Geometry: final body of the model. Coordinates: model frame, mm. Face numbers are marked on the shaded views. A direction names the side the tool comes from. Round coordinates to 2 decimals unless told otherwise and drop trailing zeros. Loops run counter-clockwise (first coordinate to the right, second up) from the corner with the lowest first, then second, coordinate; pieces in that order, holes last. Notation, with made-up numbers: (-33.75, 50.5) - (-5.75, 50.5) arc R15 ccw to (-5.75, 60.5) - close; hole circle Ø3 at (83, -27.5). An arc over 180 degrees is marked (long way). Write item = value, one per line. Start each with the question number.
Item 1: Draft query along Z for the marked faces 1, 2 and 3. Return one class per face: pulls with the +Z half, pulls with the -Z half, needs draft (parallel to the pull), parting line crosses it, or undercut.
Item 2: Access query for the marked faces 4 and 5. Directions: +Z, -Z, +X, -X, +Y, -Y. A direction counts if a zero-diameter tool reaches every point of the face in a straight line with its end or side. Return the directions, or none.
Item 3: Section C-C (z = 2.5). Return loops of the section in (x, y).
Item 4: First-contact query: pin 1 (1.5 mm diameter, centred on y = 37, z = -3.5, fed in from +X); pin 2 (6.5 mm diameter, centred on y = 15, z = 3.45, fed in from -X); pin 3 (9 mm diameter, centred on x = -5, y = 27.5, fed in from +Z); pin 4 (10 mm diameter, centred on y = 32, z = -5.5, fed in from +X). Flat tips, straight axial feed; report the tip coordinate or a pass-through.
Item 5: Section D-D (z = -0.75). Return loops of the section in (x, y), plus the area to 3 significant figures.
Item 6: Section A-A (x = 21). Return loops of the section in (y, z), plus the area to 3 significant figures.
Item 7: Line query: line 1 (Z direction, x = -17, y = 10); line 2 (Y direction, x = 3, z = 2.5); line 3 (X direction, y = 39.5, z = 6.75). Output: solid intervals per line, ascending. Write a range as from..to.
Item 8: Section B-B (y = 40). Return loops of the section in (x, z).
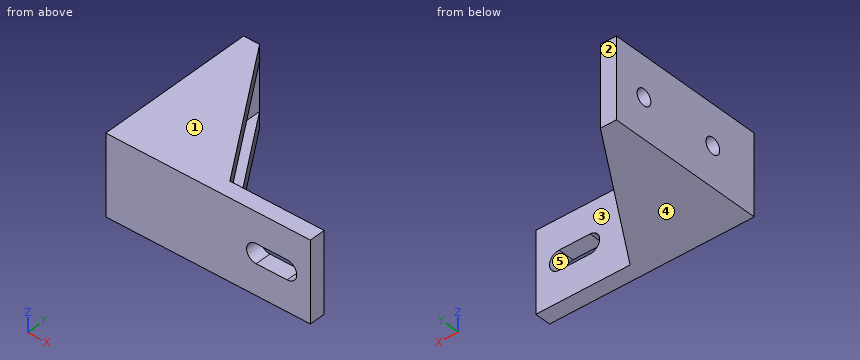
from build123d import *

# Parameters (mm, degrees)
SKETCH1_W                 = 64
SKETCH1_H                 = 15
BOSS_EXTRUDE1_DEPTH       = 5
SKETCH3_W                 = 5
SKETCH3_H                 = 15
BOSS_EXTRUDE2_DEPTH       = 45
F_5_0MM_DOWEL_HOLE1_D     = 5
F_6_0MM_DOWEL_SLOT1_DEPTH = 5
BOSS_EXTRUDE3_DEPTH       = 5
BOSS_EXTRUDE4_DEPTH       = 5


# Read off the part's stored shape, not the designer's step: Ø6.0mm Dowel Slot1
with BuildPart() as part:
    # Sketch1 → Boss-Extrude1 (new body)
    with BuildSketch(Plane(origin=(0, 0, 0), x_dir=(1, 0, 0), z_dir=(0, 1, 0))):
        with Locations((1.827783478, -3.453636176)):
            Rectangle(SKETCH1_W, SKETCH1_H)
    extrude(amount=BOSS_EXTRUDE1_DEPTH)

    # Sketch3 → Boss-Extrude2 (add)
    with BuildSketch(Plane(origin=(0, 5, 0), x_dir=(1, 0, 0), z_dir=(0, 1, 0))):
        with Locations((-27.672216522, -3.453636176)):
            Rectangle(SKETCH3_W, SKETCH3_H)
    extrude(amount=BOSS_EXTRUDE2_DEPTH)

    # Ø5.0mm Dowel Hole1 (through all)
    with Locations(Plane.ZY.offset(30.172216522)):
        with Locations((3.453636176, 15), (3.453636176, 40)):
            Hole(F_5_0MM_DOWEL_HOLE1_D / 2)

    # Ø6.0mm Dowel Slot1 outline → Ø6.0mm Dowel Slot1 (cut)
    with BuildSketch(Plane(origin=(0, 0, 0), x_dir=(1, 0, 0), z_dir=(0, 1, 0))):
        with BuildLine():
            Line((16.854220924, -6.453652479), (26.554220923, -6.453705194))
            ThreePointArc((26.554220923, -6.453705194), (29.554237227, -3.453721498), (26.554253531, -0.453705194))
            Line((26.554253531, -0.453705194), (16.854253531, -0.453652479))
            ThreePointArc((16.854253531, -0.453652479), (13.854237227, -3.453636175), (16.854220924, -6.453652479))
        make_face()
    extrude(amount=F_6_0MM_DOWEL_SLOT1_DEPTH, mode=Mode.SUBTRACT)

    # Sketch10 → Boss-Extrude3 (add)
    with BuildSketch(Plane.XY.offset(10.953636176)):
        Polygon((-25.172216522, 50), (4.327783478, 5), (33.827783478, 5), (33.827783478, 0), (-30.172216522, 0), (-30.172216522, 50), align=None)
    extrude(amount=BOSS_EXTRUDE3_DEPTH)

    # Sketch11 → Boss-Extrude4 (add)
    with BuildSketch(Plane(origin=(0, 0, -4.046363824), x_dir=(-1, 0, 0), z_dir=(0, 0, -1))):
        Polygon((25.172216522, 50), (30.172216522, 50), (30.172216522, 0), (-33.827783478, 0), (-33.827783478, 5), (-4.327783478, 5), align=None)
    extrude(amount=BOSS_EXTRUDE4_DEPTH)


solid = part.part
Taken from the geometry:
q1.face_1 = pulls with the +Z half
q1.face_2 = needs draft
q1.face_3 = undercut
q2.face_4 = -Z, +X, -X, +Y, -Y
q2.face_5 = +Y, -Y
q3.outline = (-30.17, 0) - (14.01, 0) - (14.01, 5) - (-25.17, 5) - (-25.17, 12.69) - (-30.17, 12.69) - close; (-30.17, 17.31) - (-25.17, 17.31) - (-25.17, 37.69) - (-30.17, 37.69) - close; (-30.17, 42.31) - (-25.17, 42.31) - (-25.17, 50) - (-30.17, 50) - close; (29.4, 0) - (33.83, 0) - (33.83, 5) - (29.4, 5) - close
q4.pin_1 = -16.31
q4.pin_2 = -30.17
q4.pin_3 = through
q4.pin_4 = -10.09
q5.outline = (-30.17, 0) - (33.83, 0) - (33.83, 5) - (-25.17, 5) - (-25.17, 50) - (-30.17, 50) - close
q5.area = 545 mm^2
q6.outline = (0, -9.05) - (5, -9.05) - (5, 0.45) - (0, 0.45) - close; (0, 6.45) - (5, 6.45) - (5, 15.95) - (0, 15.95) - close
q6.area = 95.0 mm^2
q7.line_1 = -9.05..-4.05, 10.95..15.95
q7.line_2 = 0..5
q7.line_3 = -30.17..-25.17
q8.outline = (-30.17, -9.05) - (-18.62, -9.05) - (-18.62, -4.05) - (-25.17, -4.05) - (-25.17, 0.95) - (-30.17, 0.95) - close; (-30.17, 5.95) - (-25.17, 5.95) - (-25.17, 10.95) - (-18.62, 10.95) - (-18.62, 15.95) - (-30.17, 15.95) - close
